Verification items for this drawing (mm, ordinates from the low corner). A direction names the side the tool comes from. Coordinates: 2 decimals unless noted, no trailing zeros. Order: outer loops, then holes, each group sorted by start corner. A loop starts at its lowest first (then second) coordinate and runs counter-clockwise, first axis right, second up. Notation, with made-up numbers: (76, 60.5) -> (87, 60.5) arc R23 ccw to (87, 82.5) -> close; hole circle Ø11 at (2.5, -1). An arc over 180 degrees is marked (long way). Write item = value, one per line. Start each with the question number.
1. Set-up check for the marked faces 1 and 2: record each of +Z, -Z, +X, -X, +Y, -Y from which the full face is reachable in a straight line by a thin tool's end or side.
2. Cross-section at A-A on z = 17. Record the cut outline in (x, y).
3. Go/stop test with a flat-tipped pin: P1, Ø1, axis at y = 0.5, z = 9.5, coming from the -X side. Record where the tip stops, or that it passes through.
4. Thickness scan on line 1 along Y through (x, z) = (3, 18.1); line 2 along Y through (x, z) = (2.05, 16.75) (1 decimal). Record the ranges inside material, lowest first. Write a range as from..to.
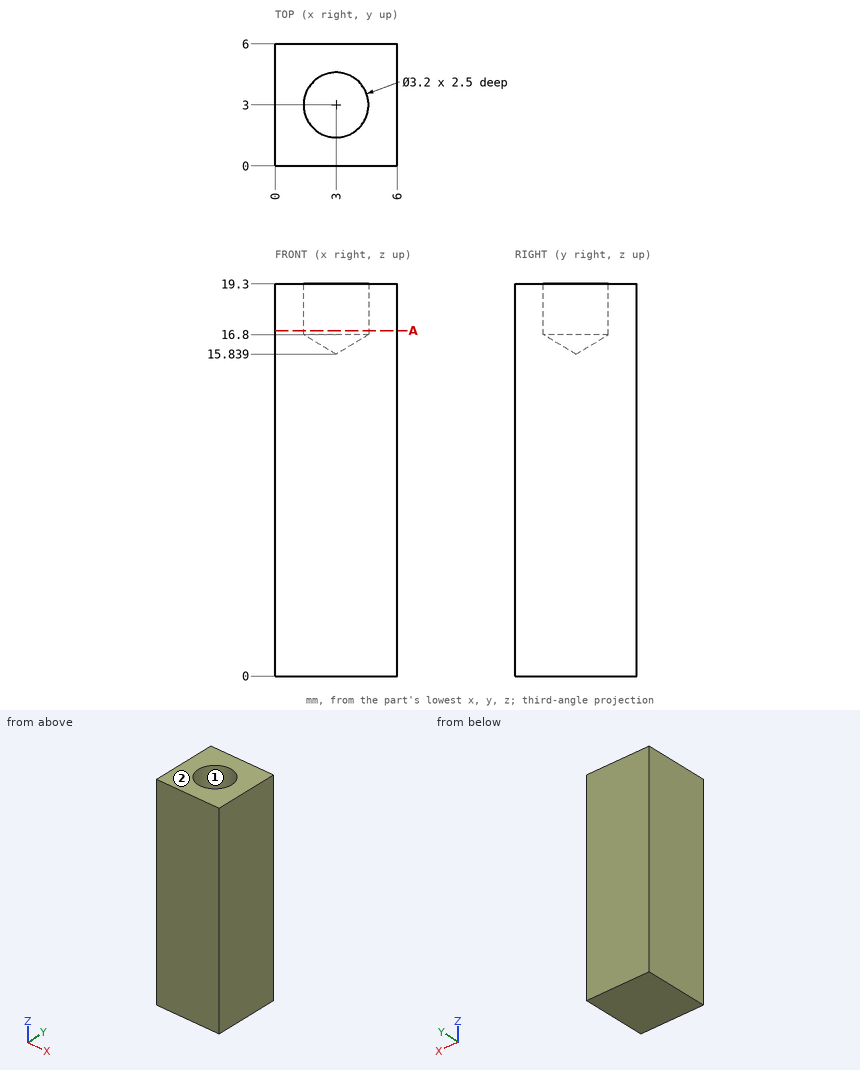
Worked out:
q1.face_1 = +Z
q1.face_2 = +Z, +X, -X, +Y, -Y
q2.outline = (0, 0) -> (6, 0) -> (6, 6) -> (0, 6) -> close; hole circle Ø3.2 at (3, 3)
q3.P1 = 0
q4.line_1 = 0..1.4, 4.6..6
q4.line_2 = 0..1.8, 4.2..6
